Design review of the part built by this model. Coordinates are the model's own, in mm. A direction names the side the tool comes from. Give positions to 0.01 mm unless a question says otherwise; leave off trailing zeros. Write each loop counter-clockwise with the first axis right and the second up, starting at its lowest first coordinate (ties: lowest second). Pieces come first, ordered by that corner, then holes. Notation, with made-up numbers: (-13, -2.5) - (17, -2.5) arc R18 ccw to (17, 17.5) - close; hole circle Ø4 at (71.5, -36). An arc over 180 degrees is marked (long way). Write each question's results on one line, items separated by ' | '. Start each with the question number.
from build123d import *

# Parameters (mm, degrees)
SKETCH1_W           = 63
SKETCH1_H           = 88
BOSS_EXTRUDE1_DEPTH = 5
SKETCH2_W           = 63
SKETCH2_H           = 5
BOSS_EXTRUDE2_DEPTH = 20
SKETCH3_R           = 1.7
CUT_EXTRUDE1_DEPTH  = 107.103722838


with BuildPart() as part:
    # Sketch1 → Boss-Extrude1 (new body)
    with BuildSketch(Plane.XY):
        with Locations((31.5, 44)):
            Rectangle(SKETCH1_W, SKETCH1_H)
    extrude(amount=BOSS_EXTRUDE1_DEPTH)

    # Sketch2 → Boss-Extrude2 (add)
    with BuildSketch(Plane(origin=(0, 0, 0), x_dir=(-1, 0, 0), z_dir=(0, 0, -1))):
        with Locations((-31.5, 2.5)):
            Rectangle(SKETCH2_W, SKETCH2_H)
    extrude(amount=BOSS_EXTRUDE2_DEPTH)

    # Sketch3 → Cut-Extrude1 (cut, through all)
    with BuildSketch(Plane(origin=(0, 5, 0), x_dir=(1, 0, 0), z_dir=(0, 1, 0))):
        with Locations(Location((51.5, 10, 0), (0, 0, 180))):
            Circle(SKETCH3_R)
        with Locations(Location((11.5, 10, 0), (0, 0, 180))):
            Circle(SKETCH3_R)
    extrude(amount=-CUT_EXTRUDE1_DEPTH, mode=Mode.SUBTRACT)


solid = part.part
Q1. Add section C-C on x = 21.5. State the section outline as (y, z) points.
Q2. Machinability: for faces 4 (the face through (32, 5, -10)), 5 (the face through (32, 3, -20)), which of the approach directions +Z, -Z, +X, -X, +Y, -Y give a long, thin tool a straight path to every point of the face, cutting with its end or side? Answer none if there is none.
Q3. The part is to be moulded in two halves that separate along X. For faces 1 (the face through (0, 34, 1)), 2 (the face through (31, 47, 0)), 3 (the face through (10.7, 2.5, -11.5)), say which applies: +X half, -X half, draft (parallel to the pull), parting line (faces both ways), or undercut.
Q4. Add section A-A on z = -10. State the section outline as (x, y) points, plus the area to 3 significant figures.
Q5. Add section D-D on y = 32. State the section outline as (x, z) points, plus the area to 3 significant figures.
Q6. For line 1 along Y through (x, z) = (37.5, -16); line 2 along Z through (x, y) = (51, 3), list the stretches that pass through material, from the lowest coordinate up. Write a range as [from, to].
Q7. Insertion check: P1, Ø3, axis at x = 35.5, y = 45, coming from the -Z side; P2, Ø1, axis at x = 40, z = -13, coming from the +Y side. Each pin has a flat end and moves straight along its axis. Give the tip position at first contact, or say it passes through.
Q8. Add section B-B on x = 11.5. State the section outline as (y, z) points, plus the area to 3 significant figures.
Result:
1) outline: (0, -20) - (5, -20) - (5, 0) - (88, 0) - (88, 5) - (0, 5) - close
2) face 4: -Z, +X, -X, +Y | face 5: -Z, +X, -X, +Y, -Y
3) face 1: -X half | face 2: draft | face 3: undercut
4) outline: (0, 0) - (9.8, 0) - (9.8, 5) - (0, 5) - close; (13.2, 0) - (49.8, 0) - (49.8, 5) - (13.2, 5) - close; (53.2, 0) - (63, 0) - (63, 5) - (53.2, 5) - close | area: 281 mm²
5) outline: (0, 0) - (63, 0) - (63, 5) - (0, 5) - close | area: 315 mm²
6) line 1: y = [0, 5] | line 2: z = [-20, -11.62], [-8.38, 5]
7) P1: stops at z = 0 | P2: stops at y = 5
8) outline: (0, -20) - (5, -20) - (5, -11.7) - (0, -11.7) - close; (0, -8.3) - (5, -8.3) - (5, 0) - (88, 0) - (88, 5) - (0, 5) - close | area: 523 mm²
